Geometry: final body of the model. Coordinates: model frame, mm. Face numbers are marked on the shaded views. A direction names the side the tool comes from. Coordinates: 2 decimals unless noted, no trailing zeros. Order: outer loops, then holes, each group sorted by start corner. A loop starts at its lowest first (then second) coordinate and runs counter-clockwise, first axis right, second up. Notation, with made-up numbers: M 51,67.25 L 93,67.25 A20 ccw 93,106.25 Z; hole C -25.5,7.25 d9. An arc over 180 degrees is marked long. One line per question, with ' | ' between items.
from build123d import *

# Parameters (mm, degrees)
BOSS_EXTRUDE1_DEPTH         = 41.275
SHELL1_START                = -34.925
SHELL1_DEPTH                = 69.85
CUT_EXTRUDE2_DEPTH          = 87.892969365
CUT_EXTRUDE2_DEPTH_BACK     = 87.892969365
SKETCH7_W                   = 6.35
SKETCH7_H                   = 3.175
SKETCH8_R                   = 3.96875
CUT_EXTRUDE3_DEPTH          = 120.685287839
F_1_4_0_25_DIAMETER_HOLE1_D = 6.35
F_1_4_0_25_DIAMETER_HOLE2_D = 6.35


# Read off the part's stored shape, not the designer's step: Shell1
with BuildPart() as part:
    # Sketch1 → Boss-Extrude1 (new, symmetric)
    with BuildSketch(Plane.XY):
        Polygon((57.15, 0), (-57.15, 0), (-57.15, 6.35), (-32.186094587, 6.35), (-28.575, 47.625), (-22.200744032, 47.625), (-21.922967525, 50.8), (21.922967525, 50.8), (22.200744032, 47.625), (28.575, 47.625), (32.186094587, 6.35), (57.15, 6.35), align=None)
    extrude(amount=BOSS_EXTRUDE1_DEPTH, both=True)

    # Shell1 outline → Shell1 (cut)
    with BuildSketch(Plane.XY.offset(SHELL1_START)):
        Polygon((26.367391632, 0), (22.756297045, 41.275), (16.382041077, 41.275), (16.10426457, 44.45), (-16.10426457, 44.45), (-16.382041077, 41.275), (-22.756297045, 41.275), (-26.367391632, 0), align=None)
    extrude(amount=SHELL1_DEPTH, mode=Mode.SUBTRACT)

    # Sketch7 → Cut-Extrude2 (cut, two sides: drawn at the far end of the back side and taken through both)
    with BuildSketch(Plane(origin=(0, 0, 0), x_dir=(0, 0, -1), z_dir=(1, 0, 0)).offset(-CUT_EXTRUDE2_DEPTH_BACK)):
        with Locations((38.1, 49.2125)):
            Rectangle(SKETCH7_W, SKETCH7_H)
    extrude(amount=CUT_EXTRUDE2_DEPTH + CUT_EXTRUDE2_DEPTH_BACK, mode=Mode.SUBTRACT)

    # Sketch8 → Cut-Extrude3 (cut, through all)
    with BuildSketch(Plane(origin=(0, 0, -50.8), x_dir=(1, 0, 0), z_dir=(0, 1, 0))):
        with Locations((44.278106598, -50.8)):
            Circle(SKETCH8_R)
        with Locations(Location((-44.278106598, -50.8, 0), (0, 0, 90))):
            Circle(SKETCH8_R)
    extrude(amount=CUT_EXTRUDE3_DEPTH, mode=Mode.SUBTRACT)

    # 1/4 (0.25) Diameter Hole1 (through all)
    with Locations(Plane(origin=(0, 50.8, 0), x_dir=(1, 0, 0), z_dir=(0, 1, 0))):
        with Locations((0, 3.175)):
            Hole(F_1_4_0_25_DIAMETER_HOLE1_D / 2)

    # 1/4 (0.25) Diameter Hole2 (through all)
    with Locations(Plane(origin=(0, 0, -41.275), x_dir=(-1, 0, 0), z_dir=(0, 0, -1))):
        with Locations((-16.382041077, 6.35), (16.382041077, 6.35)):
            Hole(F_1_4_0_25_DIAMETER_HOLE2_D / 2)


solid = part.part
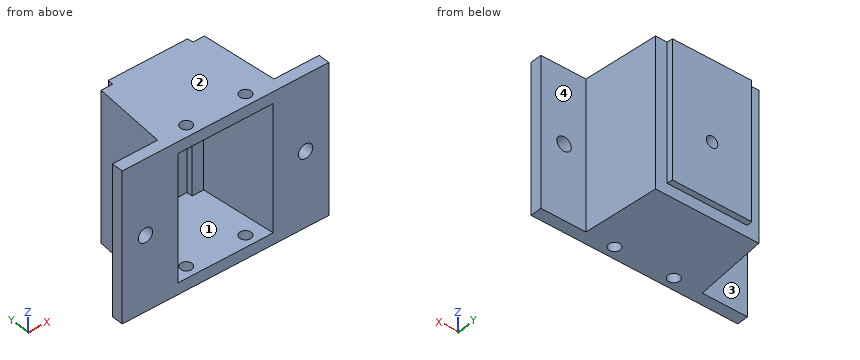
1. Section C-C, the plane y = 34. Output: boundary loops of the cut face in (x, z) (3 decimals).
Response values:
outline: M -29.767,-41.275 L 29.767,-41.275 L 29.767,41.275 L -29.767,41.275 Z; hole M -23.393,-34.925 L 23.393,-34.925 L 23.393,34.925 L -23.393,34.925 Z
2. Section D-D, the plane x = 43.5. Output: boundary loops of the cut face in (y, z) (3 decimals).
Response values:
outline: M 0,-41.275 L 6.35,-41.275 L 6.35,-3.892 L 0,-3.892 Z; M 0,3.892 L 6.35,3.892 L 6.35,41.275 L 0,41.275 Z
3. Access query for the marked faces 1, 2, 3 and 4. Directions: +Z, -Z, +X, -X, +Y, -Y. A direction counts if a zero-diameter tool reaches every point of the face in a straight line with its end or side. Return the directions, or none.
Response values:
face 1: -Y | face 2: +Z, +X, -X, +Y, -Y | face 3: +Z, -Z, -X, +Y | face 4: +Z, -Z, +X, +Y
4. Pin query (flat end, axial travel): P1, Ø4, axis at y = 16.5, z = -9, coming from the -X side; P2, Ø12, axis at y = 29, z = 25, coming from the -X side; P3, Ø12.5, axis at x = 44.28, z = 0, coming from the +Y side; P4, Ø5, axis at x = 16.38, y = 6.35, coming from the +Z side. Return the tip coordinate at first contact, or that it passes through.
Response values:
P1: stops at x = -31.47 | P2: stops at x = -30.73 | P3: stops at y = 6.35 | P4: passes through
5. Section A-A, the plane x = 0. Output: boundary loops of the cut face in (y, z) (3 decimals), and give its area (3 significant figures).
Response values:
outline: M 0,-41.275 L 47.625,-41.275 L 47.625,-34.925 L 50.8,-34.925 L 50.8,-6.35 L 44.45,-6.35 L 44.45,-34.925 L 0,-34.925 Z; M 0,34.925 L 44.45,34.925 L 44.45,0 L 50.8,0 L 50.8,41.275 L 0,41.275 Z | area: 1,030 mm^2
6. Section B-B, the plane z = -18.5. Output: boundary loops of the cut face in (x, y) (3 decimals).
Response values:
outline: M -57.15,0 L -26.367,0 L -22.756,41.275 L -16.382,41.275 L -16.104,44.45 L 16.104,44.45 L 16.382,41.275 L 22.756,41.275 L 26.367,0 L 57.15,0 L 57.15,6.35 L 32.186,6.35 L 28.575,47.625 L 22.201,47.625 L 21.923,50.8 L -21.923,50.8 L -22.201,47.625 L -28.575,47.625 L -32.186,6.35 L -57.15,6.35 Z
7. Material intervals for line 1 (X direction, y = 3.75, z = 0); line 2 (X direction, y = 3, z = 0); line 3 (Z direction, x = 24.5, y = 8) (3 decimals), sorted ascending. Write a range as [from, to].
Response values:
line 1: x = [-57.15, -48.25], [-40.31, -26.04], [26.04, 40.31], [48.25, 57.15] | line 2: x = [-57.15, -48.25], [-40.31, -26.1], [26.1, 40.31], [48.25, 57.15] | line 3: z = [-41.275, -34.925], [34.925, 41.275]
